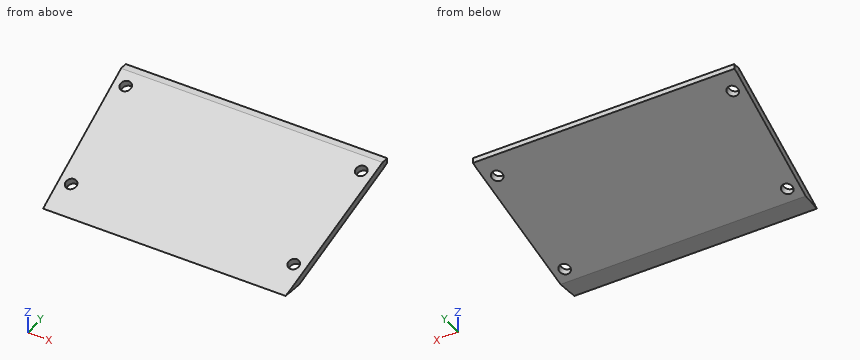
from build123d import *

# Parameters (mm, degrees)
BOSS_EXTRUDE1_DEPTH     = 1
BOSS_EXTRUDE2_REACH     = 55.976
SKETCH4_W               = 35.529511627
SKETCH4_H               = 1
CUT_EXTRUDE3_DEPTH      = 54.861211874
CUT_EXTRUDE3_DEPTH_BACK = 54.861211874
CUT_EXTRUDE4_DEPTH      = 52.541211292
CUT_EXTRUDE4_DEPTH_BACK = 52.541211292
CAVITY1_START           = -31.431872012
CAVITY1_OUTLINE_R       = 0.75
CAVITY1_DEPTH           = 1


# Read off the part's stored shape, not the designer's step: Cavity1
with BuildPart() as part:
    # Sketch1 → Boss-Extrude1 (new body)
    with BuildSketch(Plane(origin=(0, -11.283384476, 29.336799637), x_dir=(-1, 0, 0), z_dir=(0, 0.35897907930886913, -0.9333456062030595))):
        Polygon((2.285907974, 20.525558465), (-33.243603653, 20.525558465), (-32.011277476, 0.168683291), (-31.978847839, 0.168683291), (-31.978847839, -0.36702395), (1.021152161, -0.36702395), (1.021152161, 0.168683291), (1.053581797, 0.168683291), align=None)
    extrude(amount=BOSS_EXTRUDE1_DEPTH)

    # Boss-Extrude2: up to this plane
    boss_extrude2_end = Plane(origin=(160.237455752, 8.874055334, 36.705045718), z_dir=(0, -1, 0))
    # Sketch4 → Boss-Extrude2 (add, up to the surface)
    with BuildSketch(Plane(origin=(0, 19.157439808, 7.36824608), x_dir=(1, 0, 0), z_dir=(0, 0.9333456062030596, 0.35897907930886913)), mode=Mode.PRIVATE) as boss_extrude2_sk1:
        with Locations((15.47884784, -30.931872012)):
            Rectangle(SKETCH4_W, SKETCH4_H)
    boss_extrude2_tool1 = split(extrude(boss_extrude2_sk1.sketch, amount=BOSS_EXTRUDE2_REACH, mode=Mode.PRIVATE), bisect_by=boss_extrude2_end, keep=Keep.BOTH, mode=Mode.PRIVATE)
    add(boss_extrude2_tool1.solids().sort_by_distance((15.478848, 8.053545, 36.238373))[0])

    # Sketch5 → Cut-Extrude3 (cut, two sides: drawn at the far end of the back side and taken through both)
    with BuildSketch(Plane(origin=(0, 8.874055334, 0), x_dir=(1, 0, 0), z_dir=(0, 1, 0)).offset(-CUT_EXTRUDE3_DEPTH_BACK)):
        Polygon((116.276952597, -36.705045717), (33.243603653, -36.705045717), (-2.285907974, -36.705045717), (-85.319256919, -36.705045717), (-85.319256919, -202.771743607), (116.276952597, -202.771743607), align=None)
    extrude(amount=CUT_EXTRUDE3_DEPTH + CUT_EXTRUDE3_DEPTH_BACK, mode=Mode.SUBTRACT)

    # Sketch6 → Cut-Extrude4 (cut, two sides: drawn at the far end of the back side and taken through both)
    with BuildSketch(Plane(origin=(31.978847839, 0, 0), x_dir=(0, 0, -1), z_dir=(1, 0, 0)).offset(-CUT_EXTRUDE4_DEPTH_BACK)):
        Polygon((-29.205045717, -65.283704575), (-29.205045717, -11.625944667), (-29.205045717, -5.8346384), (-29.205045717, 47.823121508), (78.110474099, 47.823121508), (78.110474099, -65.283704575), align=None)
    extrude(amount=CUT_EXTRUDE4_DEPTH + CUT_EXTRUDE4_DEPTH_BACK, mode=Mode.SUBTRACT)

    # Cavity1 outline → Cavity1 (cut)
    with BuildSketch(Plane(origin=(0, 0, 0), x_dir=(1, 0, 0), z_dir=(0, 0.3589790793088689, -0.9333456062030596)).offset(CAVITY1_START)):
        with Locations((-0.531246108, -18.525558467)):
            Circle(CAVITY1_OUTLINE_R)
        with Locations((0.351610097, -3.941600191)):
            Circle(CAVITY1_OUTLINE_R)
        with Locations((30.606085582, -3.941600191)):
            Circle(CAVITY1_OUTLINE_R)
        with Locations((31.488941787, -18.525558467)):
            Circle(CAVITY1_OUTLINE_R)
    extrude(amount=CAVITY1_DEPTH, mode=Mode.SUBTRACT)


solid = part.part
The listing builds one solid part. Answer for the finished solid, in the listing's coordinates (mm). Coordinates: 2 decimals unless noted, no trailing zeros. Order: outer loops, then holes, each group sorted by start corner. A loop starts at its lowest first (then second) coordinate and runs counter-clockwise, first axis right, second up.
Q1. Given P1, Ø3, axis at y = 3, z = 33.5, coming from the -X side; P2, Ø3, axis at x = 3, y = -2.5, coming from the -Z side; P3, Ø5, axis at x = 7.5, y = 2.5, coming from the -Z side, each flat-ended and moving along its own axis, determine where each tip first touches the part or whether it passes through.
Q2. A cutting plane is placed at C-C, the plane z = 31.5. Write down the section's boundary in (x, y).
Q3. Consider line 1 (X direction, y = -9.75, z = 29.75); line 2 (Z direction, x = 16.5, y = -9.5); line 3 (Z direction, x = 1.5, y = 3.5). Determine where each line is inside the solid, lowest interval first.
Q4. A cutting plane is placed at B-B, the plane y = -3. Write down the section's boundary in (x, z).
Q5. A cutting plane is placed at A-A, the plane x = 8. Write down the section's boundary in (y, z), and give its area (3 significant figures).
Answers follow:
1. P1: stops at x = -2.03
1. P2: stops at z = 31.07
1. P3: stops at z = 32.61
2. outline: (-1.57, -2.87) - (-1.41, -5.66) - (32.37, -5.66) - (32.52, -2.87) - close
3. line 1: x = -1.14 to 32.1
3. line 2: z = 29.21 to 30.02
3. line 3: z = 33.95 to 35.02
4. outline: (-1.58, 32.52) - (-1.56, 31.45) - (32.52, 31.45) - (32.54, 32.52) - close
5. outline: (-11.63, 29.21) - (-8.84, 29.21) - (8.87, 36.02) - (8.87, 36.71) - (7.87, 36.71) - close
5. area: 20.3 mm2
